Can you work these out from the model? Positions are in its coordinate system, mm. Face numbers are marked on the shaded views. A direction names the side the tool comes from. Round coordinates to 2 decimals unless told otherwise and drop trailing zeros. Order: outer loops, then holes, each group sorted by start corner. A loop starts at its lowest first (then second) coordinate and runs counter-clockwise, first axis right, second up. Notation, with made-up numbers: (30.25, 7) -> (39.25, 7) arc R16 cw to (39.25, 22) -> close; hole circle Ø7 at (82.5, -29). An arc over 180 degrees is marked (long way). Use a Markdown table: item, result. Add a question column.
Q1. If we section it at C-C on y = 0: List the corners of the cut face in (x, z) for me, plus the area to 3 significant figures.
Q2. I'm going to push flat-ended pins straight in: pin 1 Ø8 at (x, y) = (4, -76) entering from +Z; pin 2 Ø5 at (x, y) = (-20.5, -53.5) entering from +Z; pin 3 Ø5.5 at (y, z) = (3, 6.5) entering from -X; pin 4 Ø1.5 at (x, z) = (-39, 21) entering from -Y. Where does each tip first touch, or does it pass through?
Q3. For the marked faces 1, 2, 3 and 4, which set-ups out of +Z, -Z, +X, -X, +Y, -Y let a thin tool reach every point of the face, with its end or its side?
Q4. If we section it at D-D on z = -3: List the corners of the cut face in (x, y) for me.
Q5. I need wall thicknesses on line 1 along Z through (x, y) = (71.5, 46); line 2 along Z through (x, y) = (43.5, -23.5); line 3 along Y through (x, z) = (8, 98). Which ranges of each line are inside material? Lowest first, please. Write a range as [from, to].
Q6. If we section it at B-B on z = 26: List the corners of the cut face in (x, y) for me (3 decimals).
Q7. We'd pull the mould along Y, two halves only. Please class the marked faces 5, 6 and 7: +Y half, -Y half, draft (parallel to the pull), parting line (faces both ways), or undercut.
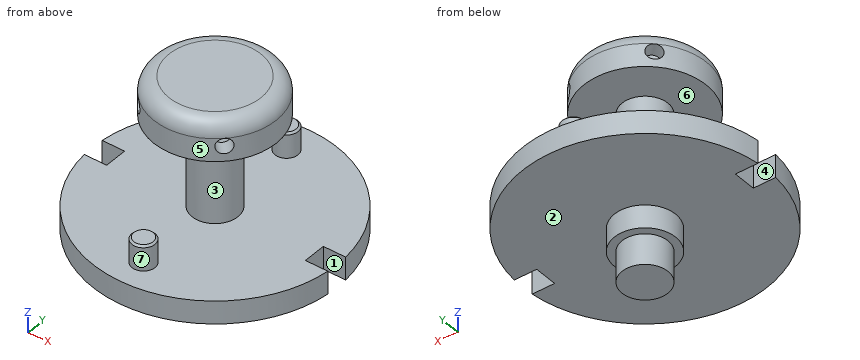
```python
from build123d import *

# Parameters (mm, degrees)
BOSS_EXTRUDE1_DEPTH = 19.05
SKETCH2_R           = 9.525
BOSS_EXTRUDE2_DEPTH = 20.828
CHAMFER1_SIZE       = 1.524
SKETCH3_R           = 19.05
BOSS_EXTRUDE3_DEPTH = 76.2
SKETCH4_R           = 25.4
BOSS_EXTRUDE4_DEPTH = 19.05
BOSS_EXTRUDE5_START = 25.4
SKETCH5_R           = 19.05
BOSS_EXTRUDE5_DEPTH = 25.4
SKETCH7_R           = 50.8
BOSS_EXTRUDE6_DEPTH = 31.75
CIRPATTERN2_COUNT   = 4
FILLET2_R           = 12.7


with BuildPart() as part:
    # Sketch1 → Boss-Extrude1 (new body)
    with BuildSketch(Plane.XY):
        with BuildLine():
            Line((101.152530245, -9.525), (82.55, -9.525))
            Line((82.55, -9.525), (82.55, 9.525))
            Line((82.55, 9.525), (101.152530245, 9.525))
            ThreePointArc((101.152530245, 9.525), (0, 101.6), (-101.152530245, 9.525))
            Line((-101.152530245, 9.525), (-82.55, 9.525))
            Line((-82.55, 9.525), (-82.55, -9.525))
            Line((-82.55, -9.525), (-101.152530245, -9.525))
            ThreePointArc((-101.152530245, -9.525), (0, -101.6), (101.152530245, -9.525))
        make_face()
    extrude(amount=BOSS_EXTRUDE1_DEPTH)

    # Sketch2 → Boss-Extrude2 (add)
    with BuildSketch(Plane.XY.offset(19.05)):
        with Locations((0, -76.2)):
            Circle(SKETCH2_R)
        with Locations(Location((0, 76.2, 0), (0, 0, 180))):
            Circle(SKETCH2_R)
    extrude(amount=BOSS_EXTRUDE2_DEPTH)

    # Chamfer1
    chamfer1_edges = [part.edges().sort_by_distance(p)[0] for p in [
        (-9.525, -76.2, 39.878),
        (9.525, 76.2, 39.878),
    ]]
    chamfer(chamfer1_edges, length=CHAMFER1_SIZE)

    # Sketch3 → Boss-Extrude3 (add)
    with BuildSketch(Plane.XY.offset(19.05)):
        with Locations(Location((0, 0, 0), (0, 0, 180))):
            Circle(SKETCH3_R)
    extrude(amount=BOSS_EXTRUDE3_DEPTH)

    # Sketch4 → Boss-Extrude4 (add)
    with BuildSketch(Plane(origin=(0, 0, 0), x_dir=(-1, 0, 0), z_dir=(0, 0, -1))):
        Circle(SKETCH4_R)
    extrude(amount=BOSS_EXTRUDE4_DEPTH)

    # Sketch5 → Boss-Extrude5 (add)
    with BuildSketch(Plane(origin=(0, 0, -19.05), x_dir=(-1, 0, 0), z_dir=(0, 0, -1)).offset(BOSS_EXTRUDE5_START)):
        Circle(SKETCH5_R)
    extrude(amount=-BOSS_EXTRUDE5_DEPTH)

    # Sketch7 → Boss-Extrude6 (add)
    with BuildSketch(Plane.XY.offset(95.25)):
        Circle(SKETCH7_R)
    extrude(amount=BOSS_EXTRUDE6_DEPTH)

    # Sketch22 → #92 (0.5) Diameter Hole1 (revolve, cut)
    with BuildSketch(Plane(origin=(35.921024484, 35.921024484, 107.95), x_dir=(-0.7071067811865464, 0.7071067811865488, 0), z_dir=(0, 0, 1))):
        Polygon((0, 0), (0, 16.002), (6.35, 12.186535069), (6.35, 0), align=None)
    f_92_0_5_diameter_hole1 = revolve(axis=Axis((40.411152545, 40.411152545, 107.95), (-0.7071067811865487, -0.7071067811865465, 0)), mode=Mode.SUBTRACT)

    # CirPattern2: #92 (0.5) Diameter Hole1 ×4 about axis
    cirpattern2_axis = Axis((0, 0, 127), (0, 0, -1))
    for i in range(1, CIRPATTERN2_COUNT):
        add(f_92_0_5_diameter_hole1.rotate(cirpattern2_axis, i * 360 / CIRPATTERN2_COUNT), mode=Mode.SUBTRACT)

    # Fillet2
    fillet2_edges = [part.edges().sort_by_distance(p)[0] for p in [
        (-50.8, 0, 127),
    ]]
    fillet(fillet2_edges, radius=FILLET2_R - 0.0001)  # a hair under: the kernel refuses the full size


solid = part.part
```
Answer below:
| question | item | result |
|---|---|---|
| 1 | outline | (-82.55, 0) -> (-25.4, 0) -> (-25.4, -19.05) -> (-19.05, -19.05) -> (-19.05, -44.45) -> (19.05, -44.45) -> (19.05, -19.05) -> (25.4, -19.05) -> (25.4, 0) -> (82.55, 0) -> (82.55, 19.05) -> (19.05, 19.05) -> (19.05, 95.25) -> (50.8, 95.25) -> (50.8, 114.3) arc R12.7 ccw to (38.1, 127) -> (-38.1, 127) arc R12.7 ccw to (-50.8, 114.3) -> (-50.8, 95.25) -> (-19.05, 95.25) -> (-19.05, 19.05) -> (-82.55, 19.05) -> close |
| 1 | area | 11,100 mm² |
| 2 | pin 1 | z = 39.88 |
| 2 | pin 2 | z = 19.05 |
| 2 | pin 3 | x = -82.55 |
| 2 | pin 4 | through |
| 3 | face 1 | +Z, -Z, +X |
| 3 | face 2 | -Z |
| 3 | face 3 | none |
| 3 | face 4 | +Z, -Z, -X |
| 4 | outline | circle Ø50.8 at (0, 0) |
| 5 | line 1 | [0, 19.05] |
| 5 | line 2 | [0, 19.05], [95.25, 120.01] |
| 5 | line 3 | [-50.17, 50.17] |
| 6 | outline | circle Ø38.1 at (0, 0); circle Ø19.05 at (0, -76.2); circle Ø19.05 at (0, 76.2) |
| 7 | face 5 | parting line |
| 7 | face 6 | draft |
| 7 | face 7 | undercut |
